Part model, mm, in its own coordinate system. A direction names the side the tool comes from. Coordinates: 2 decimals unless noted, no trailing zeros. Order: outer loops, then holes, each group sorted by start corner. A loop starts at its lowest first (then second) coordinate and runs counter-clockwise, first axis right, second up.
1) Cut at A-A (z = 0). List the corners of the cut face in (x, y), and give its area (3 significant figures).
2) Tool access for faces 4 (the flat face through (39, 0, -24)), 5 (the flat face through (0, 5, -6)): list every direction of +Z, -Z, +X, -X, +Y, -Y with a clear straight run to the whole face (end or side of a thin tool).
3) Cut at B-B (y = 0). List the corners of the cut face in (x, z).
4) Cut at D-D (z = -8). List the corners of the cut face in (x, y), and give its area (3 significant figures).
5) Pin check, flat tips, straight feed: pin 1 Ø3 at (y, z) = (12.5, 7.5) entering from -X; pin 2 Ø1.5 at (y, z) = (-16, 16) entering from -X; pin 3 Ø22 at (y, z) = (10.5, 1) entering from -X. Stop position of each tip, or through.
6) Mould opens along Z. For faces 1 (the conical face through (20.61, 15.79, -16.05)), 2 (the cylindrical face through (-3.944, -6.466, 2.681)), 3 (the flat face through (39, 22, 0)) say: +Z half, -Z half, draft (parallel to the pull), parting line (faces both ways), or undercut.
7) Wall check: L1, parallel to Y at x = 14.75, z = -16; L2, parallel to Z at x = 5, y = 16; L3, parallel to X at y = 2, z = -19. Give the ranges that are in metal, low to high.
8) Cut at C-C (y = 9.5). List the corners of the cut face in (x, z), and give its area (3 significant figures).
Solid Edge part; units mm, degrees
sketch "Sketch1" plane through (0, 0, 0) normal (1, 0, 0) x (0, 1, 0)
  line L0 (22, 24) -> (-22, 24)
  line L1 (-22, 24) -> (-22, -24)
  line L2 (-22, -24) -> (22, -24)
  line L3 (22, -24) -> (22, 24)
extrude "Extrusionsausprägung_20" add sketch "Sketch1" along normal blind 80
sketch "Sketch2" plane through (0, 0, 0) normal (-1, 0, 0) x (0, -1, 0)
  circle A0 centre (0, 0) radius 7
extrude "Extrusionsausprägung_22" add sketch "Sketch2" along normal blind 8
hole "Bohrung_4" at (0, 16, 16) direction (1, 0, 0) diameter 2.459 depth 20 tip angle 118 thread major 3 thread length 15
hole "Hole1" at (0, -16, 16) direction (1, 0, 0) diameter 2.459 depth 20 tip angle 118 thread major 3 thread length 15
hole "Hole2" at (0, -16, -16) direction (1, 0, 0) diameter 2.459 depth 20 tip angle 118 thread major 3 thread length 15
hole "Hole3" at (0, 16, -16) direction (1, 0, 0) diameter 2.459 depth 20 tip angle 118 thread major 3 thread length 15
Geometry check:
1. outline: (-8, -7) - (0, -7) - (0, -22) - (80, -22) - (80, 22) - (0, 22) - (0, 7) - (-8, 7) - close
1. area: 3,630 mm2
2. face 4: -Z, +X, -X, +Y, -Y
2. face 5: -X
3. outline: (-8, -7) - (0, -7) - (0, -24) - (80, -24) - (80, 24) - (0, 24) - (0, 7) - (-8, 7) - close
4. outline: (0, -22) - (80, -22) - (80, 22) - (0, 22) - close
4. area: 3,520 mm2
5. pin 1: stops at x = 0
5. pin 2: stops at x = 20.29
5. pin 3: stops at x = -8
6. face 1: undercut
6. face 2: parting line
6. face 3: draft
7. L1: y = -22 to -17.23, -14.77 to 14.77, 17.23 to 22
7. L2: z = -24 to -17.23, -14.77 to 14.77, 17.23 to 24
7. L3: x = 0 to 80
8. outline: (0, -24) - (80, -24) - (80, 24) - (0, 24) - close
8. area: 3,840 mm2
